```python
from build123d import *

# Parameters (mm, degrees)
SKETCH1_W               = 32.55
SKETCH1_H               = 107.3
SKETCH1_R               = 2
BOSS_EXTRUDE1_DEPTH     = 20
CUT_EXTRUDE1_DEPTH      = 35
CUT_EXTRUDE1_DEPTH_BACK = 35
CUT_EXTRUDE2_DEPTH      = 35
CUT_EXTRUDE2_DEPTH_BACK = 35
SKETCH4_R               = 4
CUT_EXTRUDE3_DEPTH      = 4
CUT_EXTRUDE4_DEPTH      = 21
CUT_EXTRUDE4_DEPTH_BACK = 21


with BuildPart() as part:
    # Sketch1 → Boss-Extrude1 (new body)
    with BuildSketch(Plane(origin=(0, 0, 0), x_dir=(1, 0, 0), z_dir=(0, 1, 0))):
        with Locations((15.875, 0)):
            Rectangle(SKETCH1_W, SKETCH1_H)
        with Locations((13.5, 47.65)):
            Circle(SKETCH1_R, mode=Mode.SUBTRACT)
    extrude(amount=BOSS_EXTRUDE1_DEPTH)

    # Sketch2 → Cut-Extrude1 (cut, two sides)
    with BuildSketch(Plane(origin=(0, 0, 0), x_dir=(0, 0, -1), z_dir=(1, 0, 0))) as cut_extrude1_sk:
        with BuildLine():
            Line((-53.65, 36.775082183), (-53.65, 15.013329403))
            ThreePointArc((-53.65, 15.013329403), (-47.333294025, 28.233294025), (-33.7, 33.6))
            Line((-33.7, 33.6), (-33.7, 36.775082183))
            Line((-33.7, 36.775082183), (-53.65, 36.775082183))
        make_face()
    extrude(amount=CUT_EXTRUDE1_DEPTH, mode=Mode.SUBTRACT)
    extrude(cut_extrude1_sk.sketch, amount=-CUT_EXTRUDE1_DEPTH_BACK, mode=Mode.SUBTRACT)

    # Sketch3 → Cut-Extrude2 (cut, two sides)
    with BuildSketch(Plane(origin=(0, 0, 0), x_dir=(0, 0, -1), z_dir=(1, 0, 0))) as cut_extrude2_sk:
        with BuildLine():
            Line((33.7, 36.775082183), (33.7, 33.6))
            ThreePointArc((33.7, 33.6), (47.333294025, 28.233294025), (53.65, 15.013329403))
            Line((53.65, 15.013329403), (53.65, 36.775082183))
            Line((53.65, 36.775082183), (33.7, 36.775082183))
        make_face()
    extrude(amount=CUT_EXTRUDE2_DEPTH, mode=Mode.SUBTRACT)
    extrude(cut_extrude2_sk.sketch, amount=-CUT_EXTRUDE2_DEPTH_BACK, mode=Mode.SUBTRACT)

    # Sketch4 → Cut-Extrude3 (cut)
    with BuildSketch(Plane(origin=(0, 20, 0), x_dir=(1, 0, 0), z_dir=(0, 1, 0))):
        with Locations((13.5, 47.65)):
            Circle(SKETCH4_R)
    extrude(amount=-CUT_EXTRUDE3_DEPTH, mode=Mode.SUBTRACT)

    # Sketch5 → Cut-Extrude4 (cut, two sides)
    with BuildSketch(Plane(origin=(0, 20, 0), x_dir=(1, 0, 0), z_dir=(0, 1, 0))) as cut_extrude4_sk:
        with BuildLine():
            Line((29.3, -27.15), (32.15, -27.15))
            Line((32.15, -27.15), (32.15, -42.15))
            Line((32.15, -42.15), (29.3, -42.15))
            ThreePointArc((29.3, -42.15), (25.3, -46.15), (29.3, -50.15))
            Line((29.3, -50.15), (32.15, -50.15))
            Line((32.15, -50.15), (32.15, -53.65))
            Line((32.15, -53.65), (50, -53.65))
            Line((50, -53.65), (50, 53.65))
            Line((50, 53.65), (32.15, 53.65))
            Line((32.15, 53.65), (32.15, 24.15))
            Line((32.15, 24.15), (29.3, 24.15))
            ThreePointArc((29.3, 24.15), (25.3, 20.15), (29.3, 16.15))
            Line((29.3, 16.15), (32.15, 16.15))
            Line((32.15, 16.15), (32.15, -18.95))
            Line((32.15, -18.95), (29.3, -18.95))
            ThreePointArc((29.3, -18.95), (25.2, -23.05), (29.3, -27.15))
        make_face()
    extrude(amount=CUT_EXTRUDE4_DEPTH, mode=Mode.SUBTRACT)
    extrude(cut_extrude4_sk.sketch, amount=-CUT_EXTRUDE4_DEPTH_BACK, mode=Mode.SUBTRACT)


solid = part.part
```
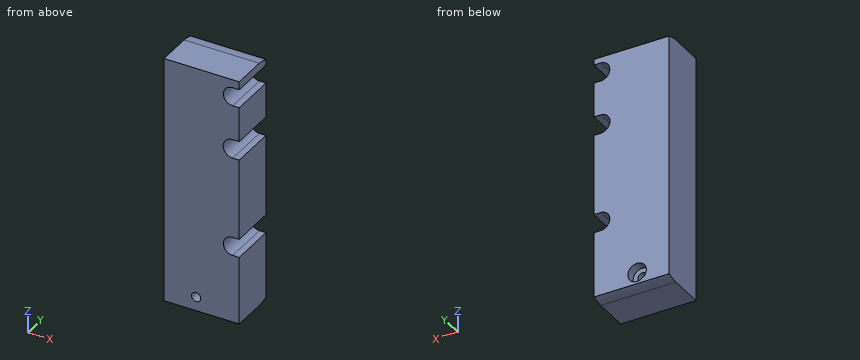
The listing builds one solid part. Answer for the finished solid, in the listing's coordinates (mm). Coordinates: 2 decimals unless noted, no trailing zeros. Loops run counter-clockwise (first coordinate to the right, second up) from the corner with the lowest first, then second, coordinate; pieces in that order, holes last. Notation, with made-up numbers: (79.25, 28) -> (103.25, 28) arc R15 ccw to (103.25, 46) -> close; hole circle Ø8 at (49.5, 33.25). An arc over 180 degrees is marked (long way). Return JSON: item names as keys, results as strings. Group by question number.
(1) Find the intervals of material crossed by probe 1 along X at (y, z) = (4.25, -47.65); probe 2 along Z at (x, y) = (31.5, 1.5); probe 3 along X at (y, z) = (18.5, -47.65), in increasing order. Write a range as from..to.
(2) A cutting plane is placed at D-D on z = -20.15. Write down the section's boundary in (x, y), and give its area (3 significant figures).
(3) A cutting plane is placed at C-C on y = 5. Write down the section's boundary in (x, z).
(4) A cutting plane is placed at B-B on z = -47.65. Write down the section's boundary in (x, y), and give its area (3 significant figures).
(5) Given pin 1 Ø3 at (y, z) = (10, -23) entering from +X; pin 2 Ø4 at (x, z) = (14, -49.5) entering from +Y, each flat-ended and moving along its own axis, determine where each tip first touches the part or whether it passes through.
(6) A cutting plane is placed at A-A on x = 13.5. Write down the section's boundary in (y, z).
The answers:
{
 "1": {"probe 1": "x = -0.4..11.5, 15.5..32.15", "probe 2": "z = -53.65..-24.15, -16.15..18.95, 27.15..42.15, 50.15..53.65", "probe 3": "x = -0.4..9.5, 17.5..32.15"},
 "2": {"outline": "(-0.4, 0) -> (25.3, 0) -> (25.3, 20) -> (-0.4, 20) -> close", "area": "514 mm^2"},
 "3": {"outline": "(-0.4, -53.65) -> (32.15, -53.65) -> (32.15, -24.15) -> (29.3, -24.15) arc R4 cw to (29.3, -16.15) -> (32.15, -16.15) -> (32.15, 18.95) -> (29.3, 18.95) arc R4.1 cw to (29.3, 27.15) -> (32.15, 27.15) -> (32.15, 42.15) -> (29.3, 42.15) arc R4 cw to (29.3, 50.15) -> (32.15, 50.15) -> (32.15, 53.65) -> (-0.4, 53.65) -> close; hole circle Ø4 at (13.5, -47.65)"},
 "4": {"outline": "(-0.4, 0) -> (11.5, 0) -> (11.5, 16) -> (9.5, 16) -> (9.5, 20) -> (-0.4, 20) -> close; (15.5, 0) -> (32.15, 0) -> (32.15, 20) -> (17.5, 20) -> (17.5, 16) -> (15.5, 16) -> close", "area": "555 mm^2"},
 "5": {"pin 1": "stops at x = 32.15", "pin 2": "stops at y = 16"},
 "6": {"outline": "(0, -53.65) -> (15.01, -53.65) arc R20 ccw to (20, -52.65) -> (20, -51.65) -> (16, -51.65) -> (16, -49.65) -> (0, -49.65) -> close; (0, -45.65) -> (16, -45.65) -> (16, -43.65) -> (20, -43.65) -> (20, 52.65) arc R20 ccw to (15.01, 53.65) -> (0, 53.65) -> close"}
}
